The drawing under review shows one solid part. Ordinate dimensions are in mm from its lowest x, y, z. A direction names the side the tool comes from. Coordinates: 2 decimals unless noted, no trailing zeros. Order: outer loops, then holes, each group sorted by start corner. A loop starts at its lowest first (then second) coordinate and runs counter-clockwise, first axis right, second up.
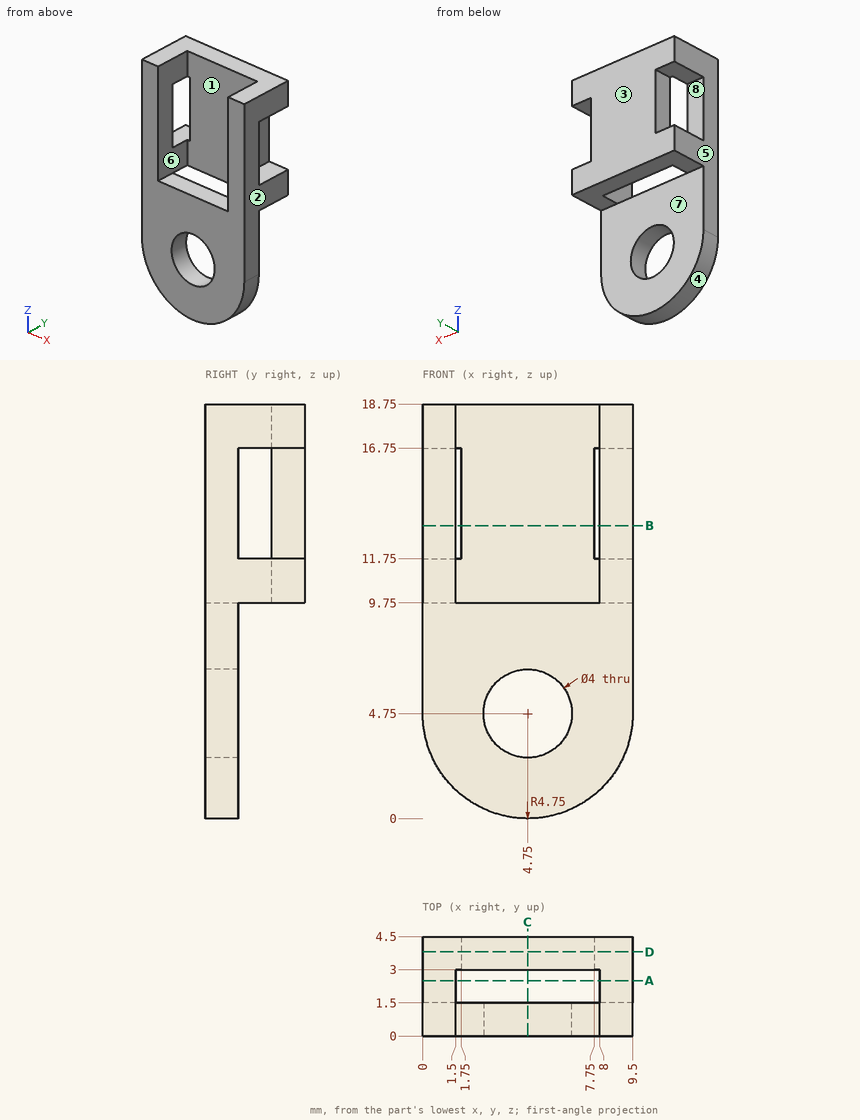
1. Take a section at A-A, the plane y = 2.5. Give the boundary of the cut face in (x, z).
Answer below:
outline: (0, 9.75) - (1.5, 9.75) - (1.5, 11.75) - (0, 11.75) - close; (0, 16.75) - (1.5, 16.75) - (1.5, 18.75) - (0, 18.75) - close; (8, 9.75) - (9.5, 9.75) - (9.5, 11.75) - (8, 11.75) - close; (8, 16.75) - (9.5, 16.75) - (9.5, 18.75) - (8, 18.75) - close
2. To check wall thickness, follow L1, parallel to X at y = 1, z = 16.5; L2, parallel to X at y = 0.65, z = 4.75; L3, parallel to Z at x = 4.75, y = 1.15. State the ranges of each line that lie inside material, in increasing order.
Answer below:
L1: x = 0 to 1.5, 8 to 9.5
L2: x = 0 to 2.75, 6.75 to 9.5
L3: z = 0 to 2.75, 6.75 to 9.75
3. Machinability: for the marked faces 4, 5, 6, 7 and 8, which of the approach directions +Z, -Z, +X, -X, +Y, -Y give a long, thin tool a straight path to every point of the face, cutting with its end or side? Answer none if there is none.
Answer below:
face 4: -Z, +Y, -Y
face 5: +Z, -Z, -X, +Y, -Y
face 6: +Z, -Y
face 7: -Z, +X, -X, +Y
face 8: +X, -X, +Y
4. The part is to be moulded in two halves that separate along X. For the marked faces 1, 2 and 3, say which applies: +X half, -X half, draft (parallel to the pull), parting line (faces both ways), or undercut.
Answer below:
face 1: undercut
face 2: +X half
face 3: draft
5. Take a section at B-B, the plane z = 13.25. Give the boundary of the cut face in (x, y).
Answer below:
outline: (0, 0) - (1.5, 0) - (1.5, 1.5) - (0, 1.5) - close; (1.75, 3) - (7.75, 3) - (7.75, 4.5) - (1.75, 4.5) - close; (8, 0) - (9.5, 0) - (9.5, 1.5) - (8, 1.5) - close
6. Clearance check with flat-ended pins moving along their axes: pin 1 Ø0.5 at (x, y) = (8.5, 3) entering from -Z; pin 2 Ø1.2 at (x, z) = (0.5, 13) entering from +Y; pin 3 Ø1.6 at (x, y) = (6.5, 1) entering from +Z; pin 4 Ø2 at (x, z) = (5.5, 4.5) entering from -Y. State where each tip first meets the part, or that it passes through.
Answer below:
pin 1: stops at z = 9.75
pin 2: stops at y = 1.5
pin 3: stops at z = 9.75
pin 4: passes through
7. Take a section at C-C, the plane x = 4.75. Give the boundary of the cut face in (y, z).
Answer below:
outline: (0, 0) - (1.5, 0) - (1.5, 2.75) - (0, 2.75) - close; (0, 6.75) - (1.5, 6.75) - (1.5, 9.75) - (0, 9.75) - close; (3, 9.75) - (4.5, 9.75) - (4.5, 18.75) - (3, 18.75) - close
8. Take a section at D-D, the plane y = 3.8. Give the boundary of the cut face in (x, z), plus the area to 3 significant figures.
Answer below:
outline: (0, 9.75) - (9.5, 9.75) - (9.5, 11.75) - (7.75, 11.75) - (7.75, 16.75) - (9.5, 16.75) - (9.5, 18.75) - (0, 18.75) - (0, 16.75) - (1.75, 16.75) - (1.75, 11.75) - (0, 11.75) - close
area: 68.0 mm2
